```python
from build123d import *

# Parameters (mm, degrees)
SKETCH1_W           = 100
SKETCH1_H           = 100
BOSS_EXTRUDE1_DEPTH = 6
CUT_EXTRUDE1_DEPTH  = 142.548578234
SKETCH3_R           = 5
CUT_EXTRUDE2_DEPTH  = 10
CUT_EXTRUDE6_DEPTH  = 142.548578234


with BuildPart() as part:
    # Sketch1 → Boss-Extrude1 (new body)
    with BuildSketch(Plane(origin=(0, 0, 0), x_dir=(1, 0, 0), z_dir=(0, 1, 0))):
        with Locations((50, -50)):
            Rectangle(SKETCH1_W, SKETCH1_H)
    extrude(amount=BOSS_EXTRUDE1_DEPTH)

    # Sketch2 → Cut-Extrude1 (cut, through all)
    with BuildSketch(Plane(origin=(0, 6, 0), x_dir=(1, 0, 0), z_dir=(0, 1, 0))):
        Polygon((48.5, 0), (51.5, 0), (51.5, -3), (53.5, -3), (53.5, -6), (51.5, -6), (51.5, -10), (48.5, -10), (48.5, -6), (46.5, -6), (46.5, -3), (48.5, -3), align=None)
        Polygon((48.5, -100), (48.5, -97), (46.5, -97), (46.5, -94), (48.5, -94), (48.5, -90), (51.5, -90), (51.5, -94), (53.5, -94), (53.5, -97), (51.5, -97), (51.5, -100), align=None)
    extrude(amount=-CUT_EXTRUDE1_DEPTH, mode=Mode.SUBTRACT)

    # Sketch3 → Cut-Extrude2 (cut)
    with BuildSketch(Plane.XZ):
        with Locations(Location((50, 50, 0), (0, 0, 270))):
            Circle(SKETCH3_R)
    extrude(amount=-CUT_EXTRUDE2_DEPTH, mode=Mode.SUBTRACT)

    # Sketch5 → Cut-Extrude6 (cut, through all)
    with BuildSketch(Plane(origin=(0, 6, 0), x_dir=(1, 0, 0), z_dir=(0, 1, 0))):
        Polygon((3, -48.5), (0, -48.5), (0, -51.5), (3, -51.5), (3, -53.5), (6, -53.5), (6, -51.5), (10, -51.5), (10, -48.5), (6, -48.5), (6, -46.5), (3, -46.5), align=None)
        Polygon((90, -48.5), (90, -51.5), (94, -51.5), (94, -53.5), (97, -53.5), (97, -51.5), (100, -51.5), (100, -48.5), (97, -48.5), (97, -46.5), (94, -46.5), (94, -48.5), align=None)
    extrude(amount=-CUT_EXTRUDE6_DEPTH, mode=Mode.SUBTRACT)


solid = part.part
```
Verification items for the finished model (mm, model axes). A direction names the side the tool comes from. Coordinates: 2 decimals unless noted, no trailing zeros. Order: outer loops, then holes, each group sorted by start corner. A loop starts at its lowest first (then second) coordinate and runs counter-clockwise, first axis right, second up. Notation, with made-up numbers: (32, 15) - (69, 15) arc R13 cw to (69, 29) - close; hole circle Ø10 at (21.25, 87). An arc over 180 degrees is marked (long way). Return JSON: item names as keys, results as strings.
(1) Thickness scan on line 1 along Z through (x, y) = (4, 4.15); line 2 along X through (y, z) = (3.05, 50); line 3 along Z through (x, y) = (90.5, 1.2). Record the ranges inside material, lowest first.
Filled sheet:
{"line 1": "z = 0 to 46.5, 53.5 to 100", "line 2": "x = 10 to 45, 55 to 90", "line 3": "z = 0 to 48.5, 51.5 to 100"}
(2) Mould release check, pull along Z, two halves, no side actions. Record for faces 1 (the flat face through (38, 0, 49)), 2 (the flat face through (50, 3, 10)), 3 (the flat face through (99, 3, 48.5)), 4 (the flat face through (92, 3, 51.5)): pulls with the +Z half, pulls with the -Z half, needs draft (parallel to the pull), parting line crosses it, or undercut.
Filled sheet:
{"face 1": "needs draft", "face 2": "pulls with the -Z half", "face 3": "undercut", "face 4": "undercut"}
(3) Section check B-B, the plane x = 50. Record the cut outline in (y, z).
Filled sheet:
{"outline": "(0, 10) - (6, 10) - (6, 45) - (0, 45) - close; (0, 55) - (6, 55) - (6, 90) - (0, 90) - close"}
(4) Access from +Z, -Z, +X, -X, +Y, -Y to the whole of each face (thin tool, end or side, straight path). Record for faces 5 (the flat face through (10, 3, 50)), 6 (the flat face through (90, 3, 50)), 7 (the flat face through (5, 3, 46.5)), 8 (the flat face through (48.5, 3, 8)), 9 (the flat face through (48.5, 3, 99)).
Filled sheet:
{"face 5": "-X, +Y, -Y", "face 6": "+X, +Y, -Y", "face 7": "+Y, -Y", "face 8": "-Z, +Y, -Y", "face 9": "+Z, +Y, -Y"}
(5) Go/stop test with a flat-tipped pin: pin 1 (1.5 mm diameter, centred on y = 2, z = 49.5, fed in from -X). Record where the tip stops, or that it passes through.
Filled sheet:
{"pin 1": "stops at x = 10"}
(6) Section check A-A, the plane z = 50. Record the cut outline in (x, y), and give its area (3 significant figures).
Filled sheet:
{"outline": "(10, 0) - (45, 0) - (45, 6) - (10, 6) - close; (55, 0) - (90, 0) - (90, 6) - (55, 6) - close", "area": "420 mm^2"}
